from build123d import *

# Parameters (mm, degrees)
BOSS_EXTRUDE1_DEPTH = 15
CHAMFER1_SIZE       = 5
CHAMFER2_SIZE       = 2
FILLET1_R           = 3
FILLET2_R           = 5


with BuildPart() as part:
    # Sketch1 → Boss-Extrude1 (new body)
    with BuildSketch(Plane(origin=(0, 0, 0), x_dir=(1, 0, 0), z_dir=(0, 1, 0))):
        Polygon((0, 0), (30, 0), (30, 15), (-30, 15), (-30, -30), (0, -30), align=None)
    extrude(amount=BOSS_EXTRUDE1_DEPTH)

    # Chamfer1
    chamfer1_edges = [part.edges().sort_by_distance(p)[0] for p in [
        (0, 0, -15),
    ]]
    chamfer(chamfer1_edges, length=CHAMFER1_SIZE)

    # Chamfer2
    chamfer2_edges = [part.edges().sort_by_distance(p)[0] for p in [
        (-30, 0, 10),
    ]]
    chamfer(chamfer2_edges, length=CHAMFER2_SIZE)

    # Fillet1
    fillet1_edges = [part.edges().sort_by_distance(p)[0] for p in [
        (0, 7.5, 30),
        (30, 7.5, 0),
        (0, 7.5, 0),
    ]]
    fillet(fillet1_edges, radius=FILLET1_R)

    # Fillet2
    fillet2_edges = [part.edges().sort_by_distance(p)[0] for p in [
        (30, 10, -15),
        (-30, 8.5, 30),
        (-30, 10, -15),
    ]]
    fillet(fillet2_edges, radius=FILLET2_R)


solid = part.part
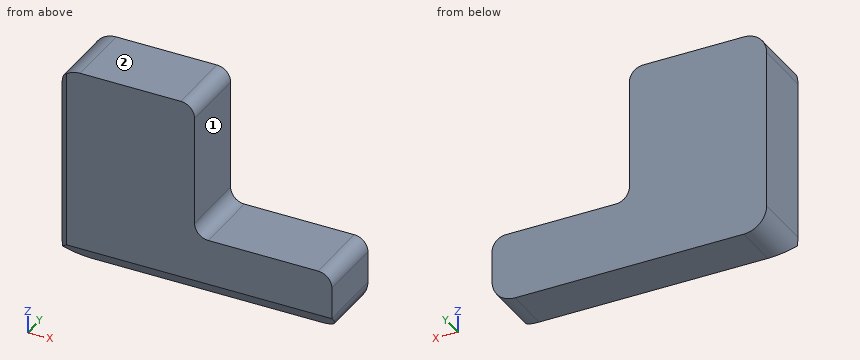
Read the model definition and answer for the solid it produces. Units are mm, in the model's axes. Face numbers are marked on the shaded views. A direction names the side the tool comes from. Round coordinates to 2 decimals unless told otherwise and drop trailing zeros. Write each loop counter-clockwise with the first axis right and the second up, starting at its lowest first coordinate (ties: lowest second). Pieces come first, ordered by that corner, then holes. Notation, with made-up numbers: (67, -40) - (84, -40) arc R9 cw to (84, -33) - close; hole circle Ø9 at (-29, 70.25). An arc over 180 degrees is marked (long way). One line per question, with ' | ' between items. Start each with the question number.
1. Section A-A (y = 8.25) is taken. Determine the outline of the cut face in (x, z).
2. Each of these flat-tipped pins is pushed along its axis until it touches: pin 1 (3 mm diameter, centred on x = 4.5, y = 3.5, fed in from +Z); pin 2 (4.5 mm diameter, centred on y = 11, z = 18, fed in from +X). Where does it stop, or does it pass through?
3. Section C-C (x = 16) is taken. Determine the outline of the cut face in (y, z), and give its area (4 significant figures).
4. Find the intervals of material crossed by probe 1 along X at (y, z) = (4, 15); probe 2 along Z at (x, y) = (9.5, 7.25); probe 3 along Y at (x, z) = (0.5, -13), in increasing order. Write a range as [from, to].
5. For the marked faces 1 and 2, determine the directions among +Z, -Z, +X, -X, +Y, -Y from which every point of the face is accessible in a straight line to the end or side of a thin tool.
6. Section B-B (z = 5.5) is taken. Determine the outline of the cut face in (x, y), and give its area (3 significant figures).
Filled in:
1) outline: (-30, -10) arc R5 ccw to (-25, -15) - (25, -15) arc R5 ccw to (30, -10) - (30, -3) arc R3 ccw to (27, 0) - (3, 0) arc R3 cw to (0, 3) - (0, 27) arc R3 ccw to (-3, 30) - (-25, 30) arc R5 ccw to (-30, 25) - close
2) pin 1: z = 0 | pin 2: x = 0
3) outline: (0, -10) - (5, -15) - (15, -15) - (15, 0) - (0, 0) - close | area: 212.5 mm²
4) probe 1: [-30, 0] | probe 2: [-15, 0] | probe 3: [3, 15]
5) face 1: +Z, +X, +Y, -Y | face 2: +Z, +X, -X, +Y, -Y
6) outline: (-30, 2) - (-28, 0) - (0, 0) - (0, 15) - (-30, 15) - close | area: 448 mm²
